Source: three-view drawing plus pictorial views. Frame: mm from the lowest corner of the part. Round coordinates to 2 decimals unless told otherwise and drop trailing zeros. Order: outer loops, then holes, each group sorted by start corner. A loop starts at its lowest first (then second) coordinate and runs counter-clockwise, first axis right, second up. Notation, with made-up numbers: (7.25, 47.5) -> (23.25, 47.5) arc R19 cw to (23.25, 77.5) -> close; hole circle Ø5 at (59.5, -0.5). An arc over 180 degrees is marked (long way). Answer as CSV lines item,"result".
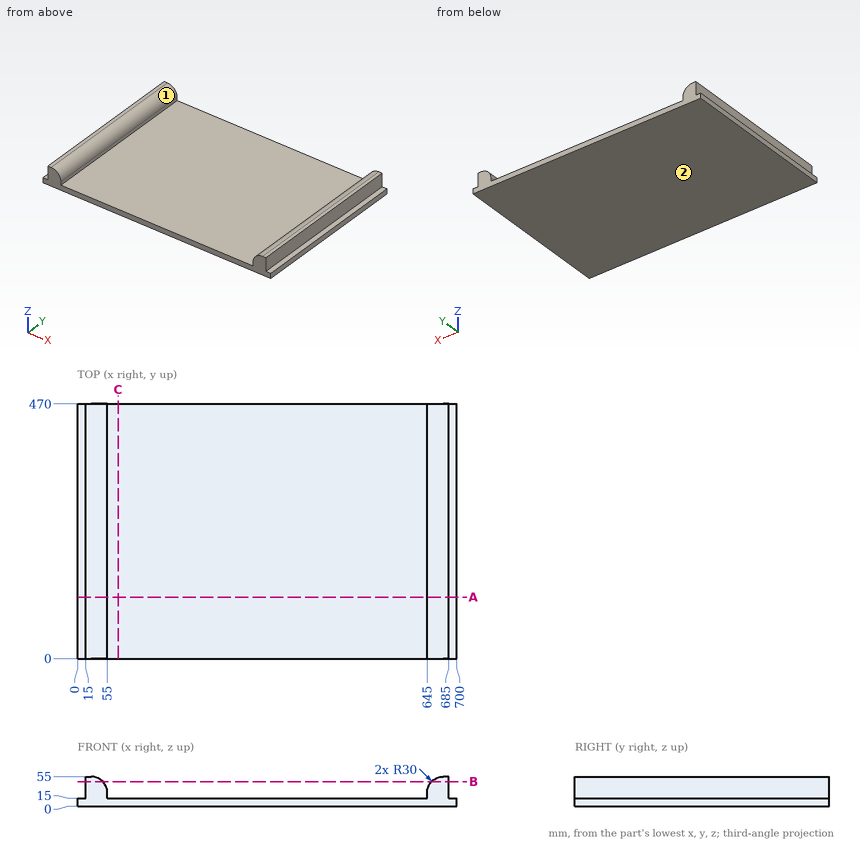
1. Section query A-A on y = 113.5. Return loops of the section in (x, z), and give its area (3 significant figures).
Results below:
outline,"(0, 0) -> (700, 0) -> (700, 15) -> (685, 15) -> (685, 55) -> (675, 55) arc R30 ccw to (645, 25) -> (645, 15) -> (55, 15) -> (55, 25) arc R30 ccw to (25, 55) -> (15, 55) -> (15, 15) -> (0, 15) -> close"
area,"13,300 mm2"
2. Section query B-B on z = 46. Return loops of the section in (x, y), and give its area (3 significant figures).
Results below:
outline,"(15, 0) -> (46.42, 0) -> (46.42, 470) -> (15, 470) -> close; (653.58, 0) -> (685, 0) -> (685, 470) -> (653.58, 470) -> close"
area,"29,500 mm2"
3. Section query C-C on x = 75. Return loops of the section in (y, z).
Results below:
outline,"(0, 0) -> (470, 0) -> (470, 15) -> (0, 15) -> close"
4. Line query: L1, parallel to X at y = 338.5, z = 17; L2, parallel to X at y = 414, z = 28; L3, parallel to Z at x = 80, y = 398. Output: solid intervals per line, ascending. Write a range as [from, to].
Results below:
L1,"[15, 55], [645, 685]"
L2,"[15, 54.85], [645.15, 685]"
L3,"[0, 15]"
5. Mould query, pull axis X, two halves, no side actions, for the marked faces 1 and 2. Classes: released by +X, released by -X, zero draft, split by the parting line, or undercut.
Results below:
face 1,"undercut"
face 2,"zero draft"
6. Pin query (flat end, axial travel): pin 1 (10 mm diameter, centred on y = 114, z = 45, fed in from -X); pin 2 (6 mm diameter, centred on y = 80.5, z = 46.5, fed in from +X); pin 3 (16.5 mm diameter, centred on x = 6.5, y = 337, fed in from +Z). Return the tip coordinate at first contact, or that it passes through.
Results below:
pin 1,"x = 15"
pin 2,"x = 685"
pin 3,"z = 15"
